Study the drawing (mm; zero at the part's minimum x, y, z) and answer. A direction names the side the tool comes from. Give positions to 0.01 mm unless a question says otherwise; leave off trailing zeros. Order: outer loops, then holes, each group sorted by start corner. A loop starts at its lowest first (then second) coordinate and runs counter-clockwise, first axis right, second up. Notation, with made-up numbers: (72.25, 36) - (98.25, 36) arc R13 cw to (98.25, 46) - close; hole circle Ø7 at (5, 86.5). An arc over 180 degrees is marked (long way). Put each result on its own line as item: value.
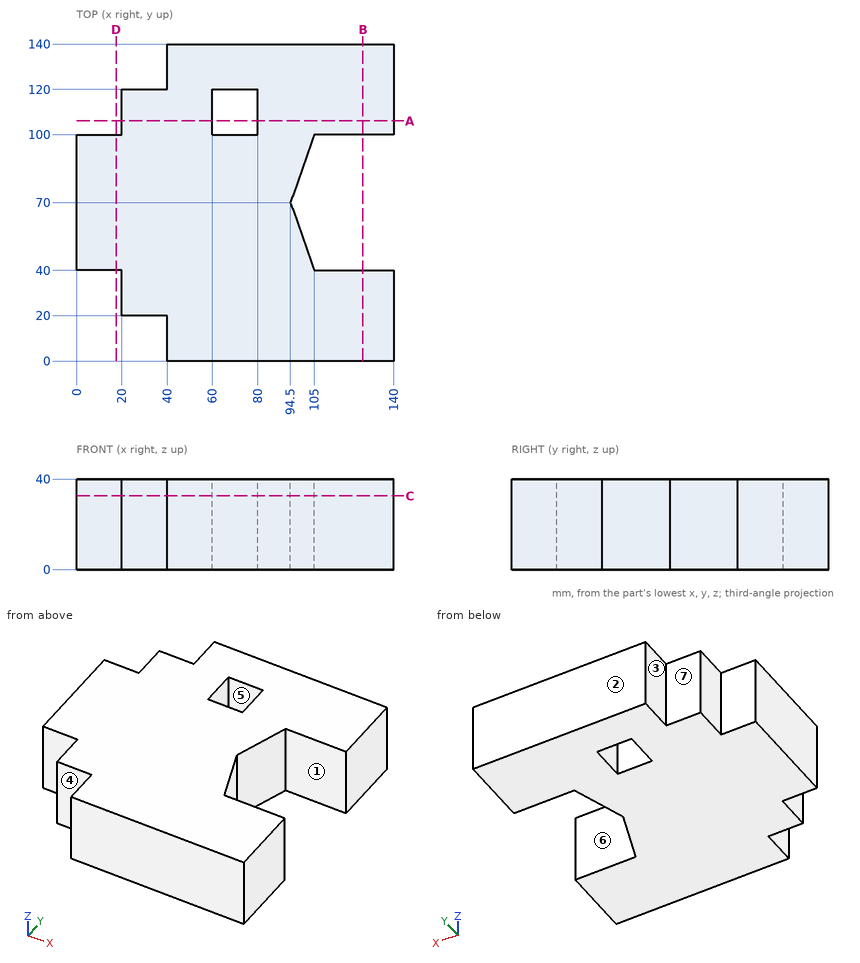
(1) Section D-D, the plane x = 17.5 is taken. Write down the section's boundary in (y, z).
Geometry check:
outline: (40, 0) - (100, 0) - (100, 40) - (40, 40) - close
(2) Section A-A, the plane y = 106 is taken. Write down the section's boundary in (x, z), then the cut area to 3 significant figures.
Geometry check:
outline: (20, 0) - (60, 0) - (60, 40) - (20, 40) - close; (80, 0) - (140, 0) - (140, 40) - (80, 40) - close
area: 4,000 mm²
(3) Section C-C, the plane z = 32.5 is taken. Write down the section's boundary in (x, y), then the cut area to 3 significant figures.
Geometry check:
outline: (0, 40) - (20, 40) - (20, 20) - (40, 20) - (40, 0) - (140, 0) - (140, 40) - (105, 40) - (94.5, 70) - (105, 100) - (140, 100) - (140, 140) - (40, 140) - (40, 120) - (20, 120) - (20, 100) - (0, 100) - close; hole (60, 100) - (80, 100) - (80, 120) - (60, 120) - close
area: 14,400 mm²
(4) Determine the mould class of the marked faces 1, 2, 3 and 4 for opening direction Y: pulls with the +Y half, pulls with the -Y half, needs draft (parallel to the pull), parting line crosses it, or undercut.
Geometry check:
face 1: undercut
face 2: pulls with the +Y half
face 3: needs draft
face 4: pulls with the -Y half
(5) Given pin 1 (16 mm diameter, centred on y = 127, z = 15, fed in from -X); pin 2 (10 mm diameter, centred on x = 29, z = 16.5, fed in from -Y); pin 3 (10 mm diameter, centred on x = 10.5, z = 19.5, fed in from +Y), each flat-ended and moving along its own axis, determine where each tip first touches the part or whether it passes through.
Geometry check:
pin 1: stops at x = 20
pin 2: stops at y = 20
pin 3: stops at y = 100
(6) Section B-B, the plane x = 126.5 is taken. Write down the section's boundary in (y, z), then the cut area to 3 significant figures.
Geometry check:
outline: (0, 0) - (40, 0) - (40, 40) - (0, 40) - close; (100, 0) - (140, 0) - (140, 40) - (100, 40) - close
area: 3,200 mm²
(7) A tool of negligible diameter and unlimited length cuts with its end or side. For the marked faces 5, 6 and 7, from which of +Z, -Z, +X, -X, +Y, -Y can it reach the whole face along a straight path? Write none if from no direction.
Geometry check:
face 5: +Z, -Z
face 6: +Z, -Z, +X
face 7: +Z, -Z, -X, +Y
(8) Straight lines are drawn through the part: line 1 (Y direction, x = 71.5, z = 25); line 2 (X direction, y = 118, z = 17.5); line 3 (Y direction, x = 112.5, z = 33.5). For each, find the intervals that lie inside material, in ascending order.
Geometry check:
line 1: y = 0 to 100, 120 to 140
line 2: x = 20 to 60, 80 to 140
line 3: y = 0 to 40, 100 to 140
